from build123d import *

# Parameters (mm, degrees)
SKETCH_1_R          = 38.5
SKETCH_1_R_2        = 27.5
EXTRUDE_1_DEPTH     = 1.25
SKETCH_3_W          = 126.6
SKETCH_3_H          = 126.6
SKETCH_3_R          = 38.5
EXTRUDE_2_DEPTH     = 2
EXTRUDE_3_REACH     = 92.022
SKETCH_4_R          = 42
SKETCH_4_R_2        = 38.5
EXTRUDE_4_DEPTH     = 1.5
SKETCH_6_W          = 5.5
SKETCH_6_H          = 1.485
EXTRUDE_5_DEPTH     = 6.43
SKETCH_7_W          = 5.5
SKETCH_7_H          = 4.5
EXTRUDE_6_DEPTH     = 4
CUT_EXTRUDE_1_DEPTH = 96.907142591
CUT_EXTRUDE_2_DEPTH = 10
EXTRUDE_7_DEPTH     = 15.08
EXTRUDE_8_DEPTH     = 1.5
EXTRUDE_9_DEPTH     = 1.5
SKETCH_17_W         = 5.5
SKETCH_17_H         = 1.485
EXTRUDE_10_DEPTH    = 6.43
SKETCH_18_W         = 5.5
SKETCH_18_H         = 4
EXTRUDE_12_DEPTH    = 4.5
CUT_EXTRUDE_3_DEPTH = 7
EXTRUDE_13_DEPTH    = 1.5
EXTRUDE_14_DEPTH    = 15.08


with BuildPart() as part:
    # Sketch 1 → Extrude 1 (new body)
    with BuildSketch(Plane(origin=(0, 0, 0), x_dir=(1, 0, 0), z_dir=(0, 1, 0))):
        with Locations(Location((0, 0, 0), (0, 0, 270))):
            Circle(SKETCH_1_R)
        with Locations(Location((0, 0, 0), (0, 0, 270))):
            Circle(SKETCH_1_R_2, mode=Mode.SUBTRACT)
    extrude(amount=EXTRUDE_1_DEPTH)


with BuildPart() as body_2:
    # Sketch 3 → Extrude 2 (new body)
    with BuildSketch(Plane(origin=(0, 7.5, 0), x_dir=(1, 0, 0), z_dir=(0, 1, 0))):
        Rectangle(SKETCH_3_W, SKETCH_3_H)
        with Locations(Location((0, 0, 0), (0, 0, 270))):
            Circle(SKETCH_3_R, mode=Mode.SUBTRACT)
    extrude(amount=EXTRUDE_2_DEPTH)

    # Sketch 4 → Extrude 3 (add, up to next)
    with BuildSketch(Plane.XZ, mode=Mode.PRIVATE) as extrude_3_sk1:
        with Locations(Location((0, 0, 0), (0, 0, 270))):
            Circle(SKETCH_4_R)
        with Locations(Location((0, 0, 0), (0, 0, 90))):
            Circle(SKETCH_4_R_2, mode=Mode.SUBTRACT)
    extrude_3_tool1 = extrude(extrude_3_sk1.sketch, amount=-EXTRUDE_3_REACH, mode=Mode.PRIVATE) - body_2.part

    add(part.part)  # Extrude 3 merges part
    add(extrude_3_tool1.solids().sort_by_distance((0, 0, 40.812061))[0])

    # Sketch 5 → Extrude 4 (add)
    with BuildSketch(Plane.XY.offset(63.3)):
        Polygon((-2.04, -22), (-2.04, -17.033321832), (2.04, -17.033321832), (2.04, -22), (7.54, -22), (7.54, 9.5), (-7.54, 9.5), (-7.54, -22), align=None)
    extrude(amount=EXTRUDE_4_DEPTH)

    # Sketch 6 → Extrude 5 (add)
    with BuildSketch(Plane(origin=(0, 0, 63.3), x_dir=(-1, 0, 0), z_dir=(0, 0, -1))):
        with Locations((-4.79, -21.2575)):
            Rectangle(SKETCH_6_W, SKETCH_6_H)
        with Locations((4.79, -21.2575)):
            Rectangle(SKETCH_6_W, SKETCH_6_H)
    extrude(amount=EXTRUDE_5_DEPTH)

    # Sketch 7 → Extrude 6 (add)
    with BuildSketch(Plane(origin=(0, 0, 56.87), x_dir=(-1, 0, 0), z_dir=(0, 0, -1))):
        with Locations((-4.79, -19.75)):
            Rectangle(SKETCH_7_W, SKETCH_7_H)
        with Locations((4.79, -19.75)):
            Rectangle(SKETCH_7_W, SKETCH_7_H)
    extrude(amount=EXTRUDE_6_DEPTH)

    # Sketch 8 → Cut-Extrude 1 (cut, through all)
    with BuildSketch(Plane(origin=(0, 9.5, 0), x_dir=(1, 0, 0), z_dir=(0, 1, 0))):
        with BuildLine():
            Line((-20, 46.775506025), (-20, 63.3))
            Line((-20, 63.3), (-63.3, 63.3))
            Line((-63.3, 63.3), (-63.3, -63.3))
            Line((-63.3, -63.3), (-20, -63.3))
            Line((-20, -63.3), (-20, -50.871877928))
            Line((-20, -50.871877928), (-20, -46.775506025))
            ThreePointArc((-20, -46.775506025), (-50.871877928, 0), (-20, 46.775506025))
        make_face()
        with BuildLine():
            Line((63.3, 63.3), (20, 63.3))
            Line((20, 63.3), (20, 46.775506025))
            ThreePointArc((20, 46.775506025), (42.458129507, 28.022405369), (50.871877928, 0))
            ThreePointArc((50.871877928, 0), (42.458129507, -28.022405369), (20, -46.775506025))
            Line((20, -46.775506025), (20, -50.871877928))
            Line((20, -50.871877928), (20, -63.3))
            Line((20, -63.3), (63.3, -63.3))
            Line((63.3, -63.3), (63.3, 63.3))
        make_face()
    extrude(amount=-CUT_EXTRUDE_1_DEPTH, mode=Mode.SUBTRACT)

    # Sketch 10 → Cut-Extrude 2 (cut)
    with BuildSketch(Plane.XZ.offset(22)):
        Polygon((5.908233118, 52.87), (7.54, 52.87), (7.54, 58.37), align=None)
        Polygon((-7.54, 58.37), (-6.0283181, 52.87), (-7.54, 52.87), align=None)
    extrude(amount=-CUT_EXTRUDE_2_DEPTH, mode=Mode.SUBTRACT)

    # Sketch 12 → Extrude 7 (add)
    with BuildSketch(Plane(origin=(7.54, 0, 0), x_dir=(0, 0, -1), z_dir=(1, 0, 0))):
        Polygon((-62.506477542, 7.5), (-63.3, 7.5), (-63.3, 6.532326517), align=None)
    extrude(amount=-EXTRUDE_7_DEPTH)

    # Sketch 14 → Extrude 8 (add)
    with BuildSketch(Plane(origin=(0, 9.5, 0), x_dir=(1, 0, 0), z_dir=(0, 1, 0))):
        Polygon((-7.54, -64.8), (-9.04, -63.3), (-7.54, -63.3), align=None)
        Polygon((7.54, -64.8), (7.54, -63.3), (9.04, -63.3), align=None)
    extrude(amount=-EXTRUDE_8_DEPTH)

    # Sketch 16 → Extrude 9 (add)
    with BuildSketch(Plane(origin=(0, 0, -63.3), x_dir=(-1, 0, 0), z_dir=(0, 0, -1))):
        Polygon((0, 9.5), (-7.54, 9.5), (-7.54, -22), (-2.04, -22), (-2.04, -17.033321832), (2.04, -17.033321832), (2.04, -22), (7.54, -22), (7.54, 9.5), align=None)
    extrude(amount=EXTRUDE_9_DEPTH)

    # Sketch 17 → Extrude 10 (add)
    with BuildSketch(Plane.XY.offset(-63.3)):
        Polygon((-7.54, -22), (-7.54, -20.5), (-2.04, -20.515), (-2.04, -22), align=None)
        with Locations((4.79, -21.2575)):
            Rectangle(SKETCH_17_W, SKETCH_17_H)
    extrude(amount=EXTRUDE_10_DEPTH)

    # Sketch 18 → Extrude 12 (add)
    with BuildSketch(Plane.XZ.offset(22)):
        with Locations((-4.79, -54.87)):
            Rectangle(SKETCH_18_W, SKETCH_18_H)
        with Locations((4.79, -54.87)):
            Rectangle(SKETCH_18_W, SKETCH_18_H)
    extrude(amount=-EXTRUDE_12_DEPTH)

    # Sketch 19 → Cut-Extrude 3 (cut)
    with BuildSketch(Plane.XZ.offset(22)):
        Polygon((-7.54, -52.87), (-7.54, -58.37), (-6.010077166, -52.87), align=None)
        Polygon((7.54, -52.87), (7.54, -58.37), (6.019440026, -52.87), align=None)
    extrude(amount=-CUT_EXTRUDE_3_DEPTH, mode=Mode.SUBTRACT)

    # Sketch 21 → Extrude 13 (add)
    with BuildSketch(Plane(origin=(0, 9.5, 0), x_dir=(1, 0, 0), z_dir=(0, 1, 0))):
        Polygon((-7.54, 64.8), (-9.04, 63.3), (-7.54, 63.3), align=None)
        Polygon((7.54, 64.8), (9.04, 63.3), (7.54, 63.3), align=None)
    extrude(amount=-EXTRUDE_13_DEPTH)

    # Sketch 23 → Extrude 14 (add)
    with BuildSketch(Plane.ZY.offset(7.54)):
        Polygon((-62.521922408, 7.5), (-63.3, 7.5), (-63.3, 6.53), align=None)
    extrude(amount=-EXTRUDE_14_DEPTH)


solid = body_2.part
Here's how the part is built. I have some questions about the finished solid (model axes, mm). A direction names the side the tool comes from. Give positions to 0.01 mm unless a question says otherwise; leave off trailing zeros. Loops run counter-clockwise (first coordinate to the right, second up) from the corner with the lowest first, then second, coordinate; pieces in that order, holes last. Notation, with made-up numbers: (8, 60) -> (33, 60) arc R31 cw to (33, 96) -> close; hole circle Ø6 at (58.5, 2). An arc over 180 degrees is marked (long way). Answer as a JSON object with one key per item and string values. Group by question number.
Item 1: I need wall thicknesses on L1, parallel to X at y = 5, z = 0; L2, parallel to X at y = 0.9, z = 0; L3, parallel to Y at x = 5.5, z = -29.5. Which ranges of each line are inside material? Lowest first, please.
Item 2: Will these pins go through, and if not, where does the flat tip stop? pin 1 (5 mm diameter, centred on x = -20, z = -27, fed in from +Y); pin 2 (3 mm diameter, centred on y = -3.5, z = -62, fed in from +X); pin 3 (10 mm diameter, centred on x = -31.5, z = 30.5, fed in from -Y).
Item 3: Thinking about a two-plate mould opening in Y: for faces 5 (the flat face through (-5, -19, -56.87)), 6 (the flat face through (-6.627, -19.782, 55.047)), 7 (the flat face through (26.14, 9.5, 28.5)), which applies, pulls with the +Y half, pulls with the -Y half, needs draft (parallel to the pull), parting line crosses it, or undercut?
Item 4: Imagine slicing it at B-B on x = 0. Write out the boundary of the cut face in (y, z).
Item 5: Imagine slicing it at C-C on y = -12.5. Write out the boundary of the cut face in (x, z), then the cut area to 3 significant figures.
Item 6: Imagine slicing it at A-A on y = 3.5. Write out the boundary of the cut face in (x, z).
Item 7: On a 3-axis mill with a long thin cutter (end or side, diameter ignored), from which of +Z, -Z, +X, -X, +Y, -Y can I reach the whole of each face in a straight line? I mean faces 1 (the cylindrical face through (12.62, 3.7, -40.06)), 2 (the flat face through (4, -17.5, 55)), 3 (the flat face through (4, -20, -52.87)), 4 (the flat face through (26.2, 1.25, -9.1)). Say none if no direction works.
Item 8: Imagine slicing it at D-D on z = -26. Write out the boundary of the cut face in (x, y).
Answer list:
{
 "1": {"L1": "x = -42 to -38.5, 38.5 to 42", "L2": "x = -42 to -27.5, 27.5 to 42", "L3": "y = 0 to 1.25"},
 "2": {"pin 1": "stops at y = 1.25", "pin 2": "stops at x = 7.54", "pin 3": "stops at y = 0"},
 "3": {"face 5": "undercut", "face 6": "needs draft", "face 7": "pulls with the +Y half"},
 "4": {"outline": "(-17.03, -64.8) -> (9.5, -64.8) -> (9.5, -38.5) -> (1.25, -38.5) -> (1.25, -27.5) -> (0, -27.5) -> (0, -42) -> (7.5, -42) -> (7.5, -62.52) -> (6.53, -63.3) -> (-17.03, -63.3) -> close; (-17.03, 63.3) -> (6.53, 63.3) -> (7.5, 62.51) -> (7.5, 42) -> (0, 42) -> (0, 27.5) -> (1.25, 27.5) -> (1.25, 38.5) -> (9.5, 38.5) -> (9.5, 64.8) -> (-17.03, 64.8) -> close"},
 "5": {"outline": "(-7.54, -64.8) -> (7.54, -64.8) -> (7.54, -63.3) -> (-7.54, -63.3) -> close; (-7.54, 63.3) -> (7.54, 63.3) -> (7.54, 64.8) -> (-7.54, 64.8) -> close", "area": "45.2 mm2"},
 "6": {"outline": "circle Ø84 at (0, 0); (-7.54, -64.8) -> (7.54, -64.8) -> (7.54, -63.3) -> (-7.54, -63.3) -> close; (-7.54, 63.3) -> (7.54, 63.3) -> (7.54, 64.8) -> (-7.54, 64.8) -> close; hole circle Ø77 at (0, 0)"},
 "7": {"face 1": "-Y", "face 2": "+X, -X", "face 3": "+X, -X, -Y", "face 4": "+Y"},
 "8": {"outline": "(-43.73, 7.5) -> (-32.98, 7.5) -> (-32.98, 0) -> (-8.96, 0) -> (-8.96, 1.25) -> (-28.39, 1.25) -> (-28.39, 9.5) -> (-43.73, 9.5) -> close; (8.96, 0) -> (32.98, 0) -> (32.98, 7.5) -> (43.73, 7.5) -> (43.73, 9.5) -> (28.39, 9.5) -> (28.39, 1.25) -> (8.96, 1.25) -> close"}
}
